from build123d import *

# Parameters (mm, degrees)
IRON_V40X40X3_1_DEPTH = 260
CUT_EXTRUDE1_DEPTH    = 10


with BuildPart() as part:
    # Sketch1 → Iron V40X40X3(1) (new body)
    with BuildSketch(Plane(origin=(0, 0, 0), x_dir=(1, 0, 0), z_dir=(0, 1, 0))):
        with BuildLine():
            Line((0, 0), (0, 40))
            ThreePointArc((0, 40), (2.121320344, 39.121320344), (3, 37))
            Line((3, 37), (3, 6.5))
            ThreePointArc((3, 6.5), (4.025126266, 4.025126266), (6.5, 3))
            Line((6.5, 3), (37, 3))
            ThreePointArc((37, 3), (39.121320344, 2.121320344), (40, 0))
            Line((40, 0), (0, 0))
        make_face()
    extrude(amount=IRON_V40X40X3_1_DEPTH)

    # Sketch2 → Cut-Extrude1 (cut)
    with BuildSketch(Plane(origin=(0, 0, 0), x_dir=(0, 0, -1), z_dir=(1, 0, 0))):
        with BuildLine():
            Line((10.5, 55), (25.5, 55))
            ThreePointArc((25.5, 55), (30.5, 50), (25.5, 45))
            Line((25.5, 45), (10.5, 45))
            ThreePointArc((10.5, 45), (5.5, 50), (10.5, 55))
        make_face()
        with BuildLine():
            Line((10.5, 85), (25.5, 85))
            ThreePointArc((25.5, 85), (30.5, 80), (25.5, 75))
            Line((25.5, 75), (10.5, 75))
            ThreePointArc((10.5, 75), (5.5, 80), (10.5, 85))
        make_face()
    extrude(amount=CUT_EXTRUDE1_DEPTH, mode=Mode.SUBTRACT)


solid = part.part
CAD build for the part. Positions are in the model's coordinates, mm. A direction names the side the tool comes from. Coordinates: 2 decimals unless noted, no trailing zeros. Order: outer loops, then holes, each group sorted by start corner. A loop starts at its lowest first (then second) coordinate and runs counter-clockwise, first axis right, second up.
Item 1: Band-saw the part on C-C on z = -33. List the corners of the cut face in (x, y).
Check sheet entries:
outline: (0, 0) - (3, 0) - (3, 260) - (0, 260) - close
Item 2: Band-saw the part on B-B on y = 80. List the corners of the cut face in (x, z), plus the area to 3 significant figures.
Check sheet entries:
outline: (0, -40) arc R3 ccw to (3, -37) - (3, -30.5) - (0, -30.5) - close; (0, -5.5) - (3.15, -5.5) arc R3.5 cw to (6.5, -3) - (37, -3) arc R3 ccw to (40, 0) - (0, 0) - close
area: 155 mm2
Item 3: Two-plate mould, pull along Y, no slides. Class faces 1 (the face through (0, 128, -20)), 2 (the face through (1.5, 80.1, -30.5)), 3 (the face through (1.6, 49.9, -5.5)), 4 (the face through (11, 260, -2)): +Y half, -Y half, draft (parallel to the pull), parting line (faces both ways), or undercut.
Check sheet entries:
face 1: draft
face 2: undercut
face 3: undercut
face 4: +Y half
Item 4: Band-saw the part on A-A on z = -14. List the corners of the cut face in (x, y).
Check sheet entries:
outline: (0, 0) - (3, 0) - (3, 45) - (0, 45) - close; (0, 55) - (3, 55) - (3, 75) - (0, 75) - close; (0, 85) - (3, 85) - (3, 260) - (0, 260) - close
Item 5: 3-axis set-ups, long thin cutter, end or side, ignore diameter. For faces 5 (the face through (20, 128, 0)), 6 (the face through (3, 128, -22)), 7 (the face through (1.5, 50.1, -30.5)): which of +Z, -Z, +X, -X, +Y, -Y reach the whole face in a straight line?
Check sheet entries:
face 5: +Z, +X, -X, +Y, -Y
face 6: -Z, +X, +Y, -Y
face 7: +X, -X
Item 6: Drill centre lines: L1, parallel to X at y = 177.5, z = -9; L2, parallel to Z at x = 19, y = 144; L3, parallel to Z at x = 38, y = 22. Where is each one in solid material? Low to high.
Check sheet entries:
L1: x = 0 to 3
L2: z = -3 to 0
L3: z = -2.83 to 0
Item 7: Pin check, flat tips, straight feed: pin 1 Ø8 at (y, z) = (144.5, -33) entering from +X; pin 2 Ø5 at (x, y) = (33.5, 74.5) entering from -Z. Stop position of each tip, or through.
Check sheet entries:
pin 1: stops at x = 3
pin 2: stops at z = -3
Item 8: Band-saw the part on D-D on x = 13.5. List the corners of the cut face in (y, z), plus the area to 3 significant figures.
Check sheet entries:
outline: (0, -3) - (260, -3) - (260, 0) - (0, 0) - close
area: 780 mm2
